Input: part model. Units: mm. Frame: model coordinates. A direction names the side the tool comes from. Coordinates: 2 decimals unless noted, no trailing zeros. Loops run counter-clockwise (first coordinate to the right, second up) from the corner with the lowest first, then second, coordinate; pieces in that order, holes last. Notation, with made-up numbers: (6, 39) -> (46, 39) arc R35 cw to (46, 74) -> close; hole circle Ø7 at (20, -23). An arc over 180 degrees is marked (long way). Put each result on its own line as item: value. Start each with the question number.
1) Cut plane B-B (y = 178). Return the cut outline in (x, z), plus the area to 3 significant figures.
2) Pull-direction query (Z, two-part tool) for faces 1 (the flat face through (-301, 286.6, -1057)), 2 (the flat face through (-301, 287.6, -1057)), 3 (the cylindrical face through (6.113, 205.588, -2048.716)); classes: pulls with the +Z half, pulls with the -Z half, needs draft (parallel to the pull), parting line crosses it, or undercut.
3) Set-up query: faces 4 (the cylindrical face through (-1066.342, -7.605, -1044.146)), 5 (the cylindrical face through (-1067.34, -7.6, -1044.12)). Return all of +Z, -Z, +X, -X, +Y, -Y with unobstructed straight access to the full face (end or side cutting, diameter ignored); none if empty.
4) Cut plane A-A (z = -1067.6). Return the cut outline in (x, y), plus the area to 3 significant figures.
5) Contact query for flat-ended pins moving along their axis: P1, Ø5, axis at y = 181.5, z = -809.5, coming from the -X side; P2, Ø10, axis at x = -662, y = 183, coming from the +Z side; P3, Ø5, axis at x = -264.5, y = 110, coming from the +Z side. Output: stop coordinate, or through.
6) Material intervals for L1, parallel to Y at x = -149, z = -1635.5; L2, parallel to Z at x = -750, y = 9; L3, parallel to Z at x = -621, y = 55.5, sorted ascending.
from build123d import *

# Parameters (mm, degrees)
SURFACE_REVOLVE1_2_ANGLE = 180
SURFACE_EXTRUDE1_3_DEPTH = 12.4
THICKEN1_T2              = 1


with BuildPart() as body_1:
    # Surface-Revolve1: a surface, the sketch's curves turned about an axis by 180 degrees
    with BuildLine(Plane(origin=(0, 0, 0), x_dir=(0, 0, -1), z_dir=(1, 0, 0)), mode=Mode.PRIVATE) as surface_revolve1_2_path:
        Line((1067.6, 287.6), (287.6, 287.6))
        ThreePointArc((287.6, 287.6), (84.236089731, 203.363910269), (0, 0))
        Line((0, 0), (0, -15))
    surface_revolve1_2 = Shell.revolve(surface_revolve1_2_path.wire(), SURFACE_REVOLVE1_2_ANGLE, Axis((0, 287.6, -1067.6), (0, -1, 0)))
    # Surface-Extrude1: a surface, the sketch's curves swept straight by 12.4 mm
    with BuildLine(Plane(origin=(0, 0, 0), x_dir=(0, 0, -1), z_dir=(1, 0, 0)), mode=Mode.PRIVATE) as surface_extrude1_3_path:
        Line((0, -15), (0, 0))
        ThreePointArc((0, 0), (84.236089731, 203.363910269), (287.6, 287.6))
        Line((287.6, 287.6), (1847.6, 287.6))
        ThreePointArc((1847.6, 287.6), (2050.963910269, 203.363910269), (2135.2, 0))
        Line((2135.2, 0), (2135.2, -15))
    surface_extrude1_3 = Shell.extrude(surface_extrude1_3_path.wire(), (1 * SURFACE_EXTRUDE1_3_DEPTH, 0 * SURFACE_EXTRUDE1_3_DEPTH, 0 * SURFACE_EXTRUDE1_3_DEPTH))
    # Surface-Knit1: the surfaces knitted into one
    surface_knit1_1 = Shell(Face.sew_faces(surface_revolve1_2.faces() + surface_extrude1_3.faces())[0])
    add(Solid.thicken(surface_knit1_1, -THICKEN1_T2))


solid = body_1.part
Results found:
1. outline: (0, -2073.5) -> (12.4, -2073.5) -> (12.4, -2072.22) -> (0, -2072.22) arc R1004.62 cw to (0, -62.98) -> (12.4, -62.98) -> (12.4, -61.7) -> (0, -61.7) arc R1005.9 ccw to start
1. area: 4,060 mm2
2. face 1: undercut
2. face 2: needs draft
2. face 3: pulls with the -Z half
3. face 4: +X, -Y
3. face 5: -X, +Y, -Y
4. outline: (-1067.6, -15) -> (-1066.6, -15) -> (-1066.6, 0) arc R286.6 cw to (-780, 286.6) -> (12.4, 286.6) -> (12.4, 287.6) -> (-780, 287.6) arc R287.6 ccw to (-1067.6, 0) -> close
4. area: 1,260 mm2
5. P1: stops at x = -971.51
5. P2: stops at z = -308.67
5. P3: stops at z = -54.63
6. L1: y = 286.6 to 287.6
6. L2: z = -1827.18 to -1825.78, -309.42 to -308.02
6. L3: z = -1929.35 to -1928.09, -207.11 to -205.85
